Input: dimensioned drawing with shaded views. Units: mm. Origin: part minimum x, y, z. Coordinates: 2 decimals unless noted, no trailing zeros. Write each loop counter-clockwise with the first axis right and the second up, starting at its lowest first coordinate (ties: lowest second). Pieces come first, ordered by that corner, then holes. Notation, with made-up numbers: M 57,50.25 L 72,50.25 A11 cw 72,67.25 Z; hole C 66,18.5 d2. An arc over 180 degrees is marked long. Use one line per item in the form item = value.
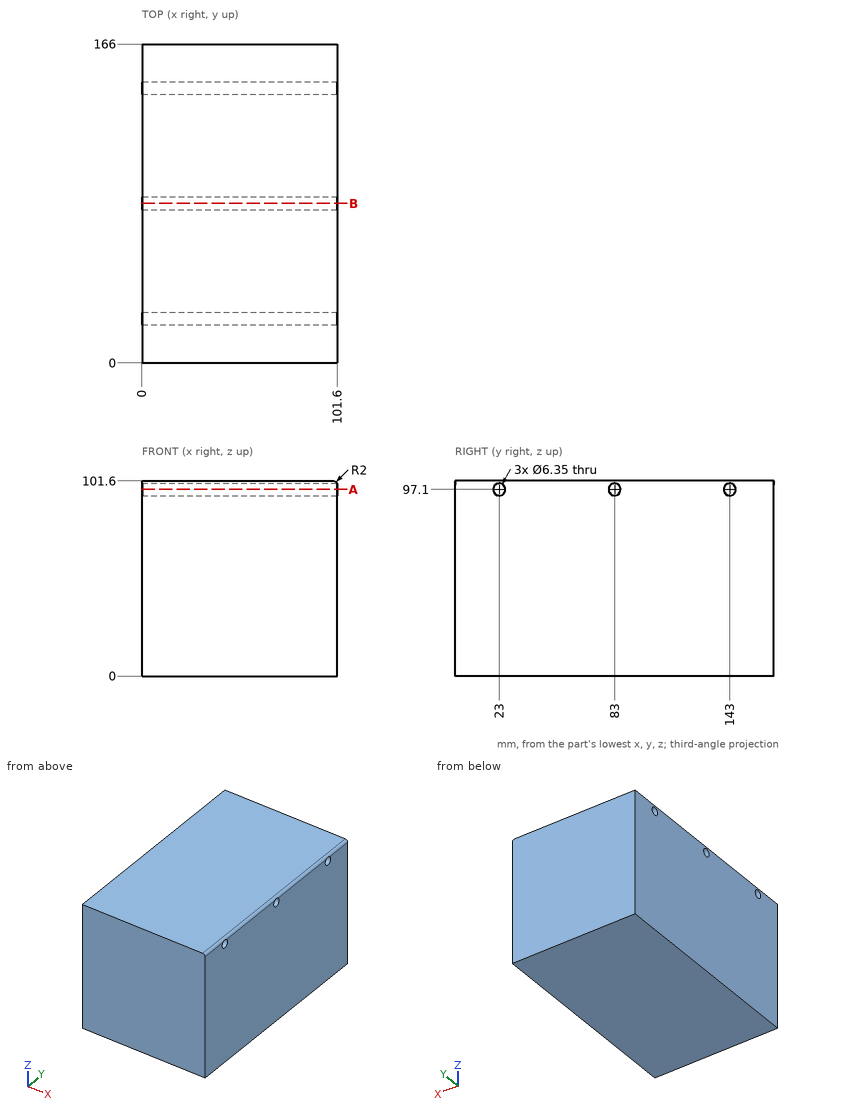
(1) Section query A-A on z = 97.1. Return the cut outline in (x, y) (3 decimals).
Computed:
outline = M 0,0 L 101.6,0 L 101.6,19.825 L 0,19.825 Z; M 0,26.175 L 101.6,26.175 L 101.6,79.825 L 0,79.825 Z; M 0,86.175 L 101.6,86.175 L 101.6,139.825 L 0,139.825 Z; M 0,146.175 L 101.6,146.175 L 101.6,166 L 0,166 Z
(2) Line query: probe 1 along Y at (x, z) = (65, 97.1) (3 decimals); probe 2 along Z at (x, y) = (72.5, 23) (3 decimals); probe 3 along Z at (x, y) = (20, 141.5). Output: solid intervals per line, ascending.
Computed:
probe_1 = 0 to 19.825, 26.175 to 79.825, 86.175 to 139.825, 146.175 to 166
probe_2 = 0 to 93.925, 100.275 to 101.6
probe_3 = 0 to 94.3, 99.9 to 101.6
(3) First-contact query: pin 1 Ø8.5 at (y, z) = (143, 97.1) entering from -X. Flat tip, straight axial feed; report the tip coordinate or a pass-through.
Computed:
pin_1 = 0
(4) Section query B-B on y = 83. Return the cut outline in (x, z) (3 decimals), plus the area to 3 significant figures.
Computed:
outline = M 0,0 L 101.6,0 L 101.6,93.925 L 0,93.925 Z; M 0,100.275 L 101.483,100.275 A2 ccw 99.6,101.6 L 0,101.6 Z
area = 9,680 mm^2
